```python
from build123d import *

# Parameters (mm, degrees)
F0_R     = 80
F1_DEPTH = 3
F2_R     = 78.8
F3_DEPTH = 25
F4_DEPTH = 1


with BuildPart() as f1:
    # F0 (on Top) → F1 (new body)
    with BuildSketch(Plane.XY):
        Circle(F0_R)
    extrude(amount=F1_DEPTH)

    # F2 (on face) → F3 (join)
    with BuildSketch(Plane.XY.offset(3)):
        Circle(F2_R)
    extrude(amount=F3_DEPTH)

    # F4 (add): a face of the model
    f4_faces = [f1.faces().sort_by_distance(p)[0] for p in [
        (0, 0, 0),
    ]]
    extrude(f4_faces, amount=F4_DEPTH)


solid = f1.part
```
Input: part model. Units: mm. Frame: model coordinates. A direction names the side the tool comes from. Coordinates: 2 decimals unless noted, no trailing zeros. Write each loop counter-clockwise with the first axis right and the second up, starting at its lowest first coordinate (ties: lowest second). Pieces come first, ordered by that corner, then holes. Notation, with made-up numbers: (-10.5, 24) - (11.5, 24) arc R10 cw to (11.5, 41) - close; hole circle Ø11 at (88, -24). An arc over 180 degrees is marked (long way). Put each result on its own line as item: value. Start each with the question number.
1) Ray query, L1, parallel to Z at x = 46, y = 65; L2, parallel to X at y = 2.5, z = 13; L3, parallel to X at y = 24.5, z = 21.25. Return the intervals inside material, ascending.
2) Contact query for flat-ended pins moving along their axis: pin 1 (12 mm diameter, centred on y = -12.5, z = 5, fed in from -X); pin 2 (1 mm diameter, centred on x = 2.5, z = 15.5, fed in from -Y); pin 3 (1.5 mm diameter, centred on y = 22, z = 2, fed in from -X); pin 4 (6 mm diameter, centred on x = -58.5, y = -63, fed in from +Z). Output: stop coordinate, or through.
3) Reachability of faces 1 (the face through (-62.53, -47.95, 15.32)), 2 (the face through (-1, 1, -1)) from +Z, -Z, +X, -X, +Y, -Y: full face, straight path, thin tool, end or side. Return the list, or none.
4) Cut plane C-C (y = 6.5). Return the cut outline in (x, z).
5) Cut plane A-A (x = -61). Return the cut outline in (y, z), plus the area to 3 significant figures.
6) Cut plane B-B (z = 9.25). Return the cut outline in (x, y), plus the area to 3 significant figures.
Resolved:
1. L1: z = -1 to 3
1. L2: x = -78.76 to 78.76
1. L3: x = -74.89 to 74.89
2. pin 1: stops at x = -79.71
2. pin 2: stops at y = -78.77
2. pin 3: stops at x = -77.13
2. pin 4: passes through
3. face 1: +Z
3. face 2: -Z, +X, -X, +Y, -Y
4. outline: (-79.74, -1) - (79.74, -1) - (79.74, 3) - (78.53, 3) - (78.53, 28) - (-78.53, 28) - (-78.53, 3) - (-79.74, 3) - close
5. outline: (-51.76, -1) - (51.76, -1) - (51.76, 3) - (49.88, 3) - (49.88, 28) - (-49.88, 28) - (-49.88, 3) - (-51.76, 3) - close
5. area: 2,910 mm2
6. outline: circle Ø157.6 at (0, 0)
6. area: 19,500 mm2
